Could you check a few things on this model? Use its own coordinates, in mm. Give positions to 0.01 mm unless a question says otherwise; leave off trailing zeros. Loops run counter-clockwise (first coordinate to the right, second up) from the corner with the lowest first, then second, coordinate; pieces in that order, holes last. Notation, with made-up numbers: (34, 22.25) -> (45, 22.25) arc R25 ccw to (45, 38.25) -> close; hole circle Ø8 at (45, -1). An arc over 180 degrees is marked (long way). Put each result on its own line as item: value.
```python
from build123d import *

# Parameters (mm, degrees)
F0_W     = 43
F0_H     = 46
F0_R     = 4.025
F0_R_2   = 11.5
F0_H_2   = 3.15
F1_DEPTH = 5
F2_R     = 5


# Not quite as in the source:
# - ends of sketch curves that miss each other by under 0.0002 mm in the source are joined


with BuildPart() as f1:
    # F0 (on Top) → F1 (new body)
    with BuildSketch(Plane.XY):
        Polygon((-21.5, -23), (-21.5, 23), (-31.8, 23), (-31.8, -26.15), (-21.5, -26.15), align=None)
        with BuildLine():
            ThreePointArc((-23.5, -16.35), (-25.15, -18), (-26.8, -16.35))
            Line((-26.8, -16.35), (-26.8, -14.75))
            ThreePointArc((-26.8, -14.75), (-25.15, -13.1), (-23.5, -14.75))
            Line((-23.5, -14.75), (-23.5, -16.35))
        make_face(mode=Mode.SUBTRACT)
        with BuildLine():
            ThreePointArc((-23.5, 14.75), (-25.15, 13.1), (-26.8, 14.75))
            Line((-26.8, 14.75), (-26.8, 16.35))
            ThreePointArc((-26.8, 16.35), (-25.15, 18), (-23.5, 16.35))
            Line((-23.5, 16.35), (-23.5, 14.75))
        make_face(mode=Mode.SUBTRACT)
        Rectangle(F0_W, F0_H)
        with BuildLine():
            ThreePointArc((-13.2000083949, -16.3447366346), (-13.2000020987, -16.3473683139), (-13.2, -16.35))
            ThreePointArc((-13.2, -16.35), (-14.85, -18), (-16.5, -16.35))
            Line((-16.5, -16.35), (-16.5, -14.75))
            ThreePointArc((-16.5, -14.75), (-14.8526316861, -13.1000020987), (-13.2000083949, -14.7447366346))
            ThreePointArc((-13.2000083949, -14.7447366346), (-13.2000020987, -14.7473683139), (-13.2, -14.75))
            Line((-13.2, -14.75), (-13.2000083949, -16.3447366346))
        make_face(mode=Mode.SUBTRACT)
        with Locations((0, -17.125)):
            Circle(F0_R, mode=Mode.SUBTRACT)
        with BuildLine():
            ThreePointArc((16.5, -16.35), (14.85, -18), (13.2, -16.35))
            Line((13.2, -16.35), (13.2, -14.75))
            ThreePointArc((13.2, -14.75), (14.85, -13.1), (16.5, -14.75))
            Line((16.5, -14.75), (16.5, -16.35))
        make_face(mode=Mode.SUBTRACT)
        with BuildLine():
            ThreePointArc((-16.5, 16.35), (-14.85, 18), (-13.2, 16.35))
            Line((-13.2, 16.35), (-13.2, 14.75))
            ThreePointArc((-13.2, 14.75), (-14.85, 13.1), (-16.5, 14.75))
            Line((-16.5, 14.75), (-16.5, 16.35))
        make_face(mode=Mode.SUBTRACT)
        Circle(F0_R_2, mode=Mode.SUBTRACT)
        with BuildLine():
            ThreePointArc((13.2, 16.35), (14.85, 18), (16.5, 16.35))
            ThreePointArc((16.5, 16.35), (16.4999973784, 16.347058674), (16.4999895135, 16.3441173573))
            Line((16.4999895135, 16.3441173573), (16.4999895135, 14.75))
            ThreePointArc((16.4999895135, 14.75), (14.85, 13.1), (13.2, 14.75))
            Line((13.2, 14.75), (13.2, 16.35))
        make_face(mode=Mode.SUBTRACT)
        with Locations((0, -24.575)):
            Rectangle(F0_W, F0_H_2)
        Polygon((31.7999895135, 23), (21.5, 23), (21.5, -23), (21.5, -26.15), (31.7999895135, -26.15), align=None)
        with BuildLine():
            ThreePointArc((26.8, -16.35), (25.15, -18), (23.5, -16.35))
            Line((23.5, -16.35), (23.5, -14.75))
            ThreePointArc((23.5, -14.75), (25.15, -13.1), (26.8, -14.75))
            Line((26.8, -14.75), (26.8, -16.35))
        make_face(mode=Mode.SUBTRACT)
        with BuildLine():
            ThreePointArc((26.7999895135, 14.75), (25.1499895135, 13.1), (23.4999895135, 14.75))
            Line((23.4999895135, 14.75), (23.4999895135, 16.3441173573))
            ThreePointArc((23.4999895135, 16.3441173573), (25.1499895135, 17.9941173573), (26.7999895135, 16.3441173573))
            Line((26.7999895135, 16.3441173573), (26.7999895135, 14.75))
        make_face(mode=Mode.SUBTRACT)
    extrude(amount=F1_DEPTH)

    # F2
    f2_edges = [f1.edges().sort_by_distance(p)[0] for p in [
        (-31.8, 23, 2.5),
        (-31.8, -26.15, 2.5),
        (31.79999, -26.15, 2.5),
        (31.79999, 23, 2.5),
    ]]
    fillet(f2_edges, radius=F2_R)


solid = f1.part
```
1. If we section it at D-D (x = 14.85): List the corners of the cut face in (y, z) for me.
Recorded:
outline: (-26.15, 0) -> (-18, 0) -> (-18, 5) -> (-26.15, 5) -> close; (-13.1, 0) -> (13.1, 0) -> (13.1, 5) -> (-13.1, 5) -> close; (18, 0) -> (23, 0) -> (23, 5) -> (18, 5) -> close
2. If we section it at B-B (x = 0): List the corners of the cut face in (y, z) for me, then the cut area to 3 significant figures.
Recorded:
outline: (-26.15, 0) -> (-21.15, 0) -> (-21.15, 5) -> (-26.15, 5) -> close; (-13.1, 0) -> (-11.5, 0) -> (-11.5, 5) -> (-13.1, 5) -> close; (11.5, 0) -> (23, 0) -> (23, 5) -> (11.5, 5) -> close
area: 90.5 mm^2
3. If we section it at A-A (y = 0): List the corners of the cut face in (x, z) for me.
Recorded:
outline: (-31.8, 0) -> (-11.5, 0) -> (-11.5, 5) -> (-31.8, 5) -> close; (11.5, 0) -> (31.8, 0) -> (31.8, 5) -> (11.5, 5) -> close
4. I need wall thicknesses on line 1 (Y direction, x = 0, z = 1.8); line 2 (X direction, y = 15.5, z = 4); line 3 (Y direction, x = -1.5, z = 1.7). Which ranges of each line are inside material? Lowest first, please.
Recorded:
line 1: y = -26.15 to -21.15, -13.1 to -11.5, 11.5 to 23
line 2: x = -31.8 to -26.8, -23.5 to -16.5, -13.2 to 13.2, 16.5 to 23.5, 26.8 to 31.8
line 3: y = -26.15 to -20.86, -13.39 to -11.4, 11.4 to 23
5. Thinking about a two-plate mould opening in X: for faces 1 (the face through (0, -12, 0)), 2 (the face through (13.2, -16, 2)), 3 (the face through (31.8, -2, 2)), which applies, pulls with the +X half, pulls with the -X half, needs draft (parallel to the pull), parting line crosses it, or undercut?
Recorded:
face 1: needs draft
face 2: undercut
face 3: pulls with the +X half
6. If we section it at C-C (y = -5): List the corners of the cut face in (x, z) for me, then the cut area to 3 significant figures.
Recorded:
outline: (-31.8, 0) -> (-10.36, 0) -> (-10.36, 5) -> (-31.8, 5) -> close; (10.36, 0) -> (31.8, 0) -> (31.8, 5) -> (10.36, 5) -> close
area: 214 mm^2
